```python
from build123d import *

# Parameters (mm, degrees)
SKETCH_R      = 25.4
SKETCH_R_2    = 19.05
SKETCH_R_3    = 12.7
SKETCH_W      = 6
SKETCH_H      = 2
PAD_DEPTH     = 1.7
SKETCH001_W   = 1.720414
SKETCH001_H   = 4.989207
SKETCH001_W_2 = 2.270946
POCKET_DEPTH  = 5


with BuildPart() as part:
    # Sketch → Pad (new body)
    with BuildSketch(Plane.XY):
        with BuildLine():
            Line((-2.4, 19.353417), (-2.4, 17.852674))
            Line((-2.4, 17.852674), (-18.357101, 17.852674))
            ThreePointArc((-18.357101, 17.852674), (-48.5501, 15.352674), (-18.357101, 12.852674))
            Line((-18.357101, 12.852674), (-2.4, 12.852674))
            Line((-2.4, 12.852674), (-2.4, 0))
            Line((-2.4, 0), (2.4, 0))
            Line((2.4, 0), (2.4, 12.852674))
            Line((2.4, 12.852674), (20.245403, 12.852674))
            ThreePointArc((20.245403, 12.852674), (63.1999, 15.352674), (20.245403, 17.852674))
            Line((20.245403, 17.852674), (2.4, 17.852674))
            Line((2.4, 17.852674), (2.4, 19.353417))
            ThreePointArc((2.4, 19.353417), (0, 75.05), (-2.4, 19.353417))
        make_face()
        with Locations((0, 47.15)):
            Circle(SKETCH_R, mode=Mode.SUBTRACT)
        with Locations((41.6499, 15.352674)):
            Circle(SKETCH_R_2, mode=Mode.SUBTRACT)
        with Locations((-33.3501, 15.352674)):
            Circle(SKETCH_R_3, mode=Mode.SUBTRACT)
        with Locations((0, 6)):
            Rectangle(SKETCH_W, SKETCH_H)
    extrude(amount=PAD_DEPTH)

    # Sketch001 (on Face25 of Pad) → Pocket (cut)
    with BuildSketch(Plane.XY.offset(1.7)):
        with Locations((-2.723439, 2.494603)):
            Rectangle(SKETCH001_W, SKETCH001_H)
        with Locations((3.02274, 2.494603)):
            Rectangle(SKETCH001_W_2, SKETCH001_H)
    extrude(amount=-POCKET_DEPTH, mode=Mode.SUBTRACT)


solid = part.part
```
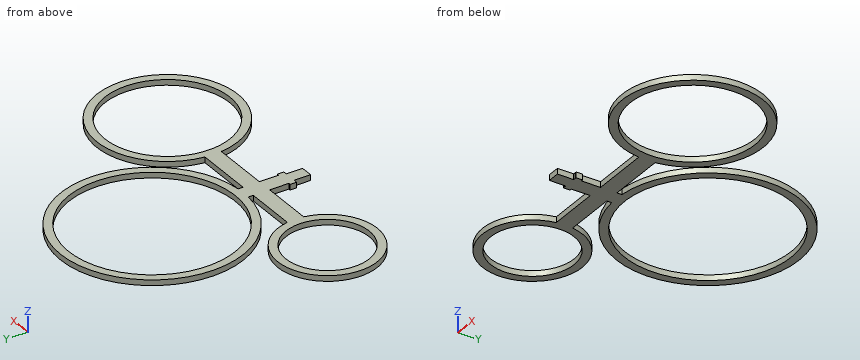
Geometry: final body of the model. Coordinates: model frame, mm. Round coordinates to 2 decimals unless told otherwise and drop trailing zeros. Loops run counter-clockwise (first coordinate to the right, second up) from the corner with the lowest first, then second, coordinate; pieces in that order, holes last.
Item 1: Line query: L1, parallel to X at y = 24, z = 1.3; L2, parallel to Y at x = -12.5, z = 0.35; L3, parallel to Y at x = -3.5, z = 0.85. Output: solid intervals per line, ascending.
Checked values:
L1: x = -45.85 to -42.65, -24.05 to -20.85, -15.57 to -10.45, 10.45 to 15.57, 21.91 to 24.68, 58.62 to 61.39
L2: y = 12.85 to 17.85, 22.21 to 25.04, 69.26 to 72.09
L3: y = 12.85 to 17.85, 19.47 to 21.99, 72.31 to 74.83
Item 2: Section C-C, the plane x = 16.5. Output: boundary loops of the cut face in (y, z), plus the area to 3 significant figures.
Checked values:
outline: (12.85, 0) - (17.85, 0) - (17.85, 1.7) - (12.85, 1.7) - close; (24.65, 0) - (27.84, 0) - (27.84, 1.7) - (24.65, 1.7) - close; (66.46, 0) - (69.65, 0) - (69.65, 1.7) - (66.46, 1.7) - close
area: 19.3 mm2
Item 3: Contact query for flat-ended pins moving along their axis: P1, Ø0.5, axis at y = 6, z = 1, coming from the +X side; P2, Ø1, axis at x = 50.5, z = 1, coming from the +Y side; P3, Ø0.5, axis at x = 2.5, z = 1, coming from the -Y side. Output: stop coordinate, or through.
Checked values:
P1: stops at x = 61.18
P2: stops at y = 35.22
P3: stops at y = 4.99
Item 4: Section B-B, the plane y = 47.15. Output: boundary loops of the cut face in (x, z).
Checked values:
outline: (-27.9, 0) - (-25.4, 0) - (-25.4, 1.7) - (-27.9, 1.7) - close; (25.4, 0) - (27.9, 0) - (27.9, 1.7) - (25.4, 1.7) - close
Item 5: Section A-A, the plane x = 0. Output: boundary loops of the cut face in (y, z).
Checked values:
outline: (0, 0) - (21.75, 0) - (21.75, 1.7) - (0, 1.7) - close; (72.55, 0) - (75.05, 0) - (75.05, 1.7) - (72.55, 1.7) - close
Item 6: Section D-D, the plane z = 0.75. State how many separate pieces and enclosed holes the cut face has, plus the area to 3 significant figures.
Checked values:
separate pieces: 1
enclosed holes: 3
area: 1,210 mm2
